Source: three-view drawing plus pictorial views. Frame: mm from the lowest corner of the part. A direction names the side the tool comes from. Give positions to 0.01 mm unless a question says otherwise; leave off trailing zeros. Write each loop counter-clockwise with the first axis right and the second up, starting at its lowest first coordinate (ties: lowest second). Pieces come first, ordered by that corner, then holes.
Q1. Pin query (flat end, axial travel): pin 1 (2.5 mm diameter, centred on x = 3.05, y = 4.5, fed in from +Z); pin 2 (3 mm diameter, centred on x = 13.5, y = 5, fed in from +Z); pin 3 (0.9 mm diameter, centred on x = 17, y = 6, fed in from -Z); pin 4 (1 mm diameter, centred on y = 3.5, z = 5.5, fed in from -X). Return the tip coordinate at first contact, or that it passes through.
Q2. Line query: L1, parallel to Y at x = 9, z = 4.2; L2, parallel to X at y = 3, z = 4.25; L3, parallel to Y at x = 12.25, z = 0.5. Output: solid intervals per line, ascending.
Q3. Cut plane B-B on z = 1.75. Return the cut outline in (x, y), plus the area to 3 significant figures.
Q4. Cut plane A-A on y = 4.5. Return the cut outline in (x, z), plus the area to 3 significant figures.
Q5. Cut plane D-D on x = 12.5. Return the cut outline in (y, z).
Q6. Draft query along Y for the marked faces 4, 5, 6 and 7. Return one class per face: pulls with the +Y half, pulls with the -Y half, needs draft (parallel to the pull), parting line crosses it, or undercut.
Q7. Cut plane C-C on y = 6. Return the cut outline in (x, z).
Q8. Reachability of the marked faces 1, 2 and 3 from +Z, -Z, +X, -X, +Y, -Y: full face, straight path, thin tool, end or side. Return the list, or none.
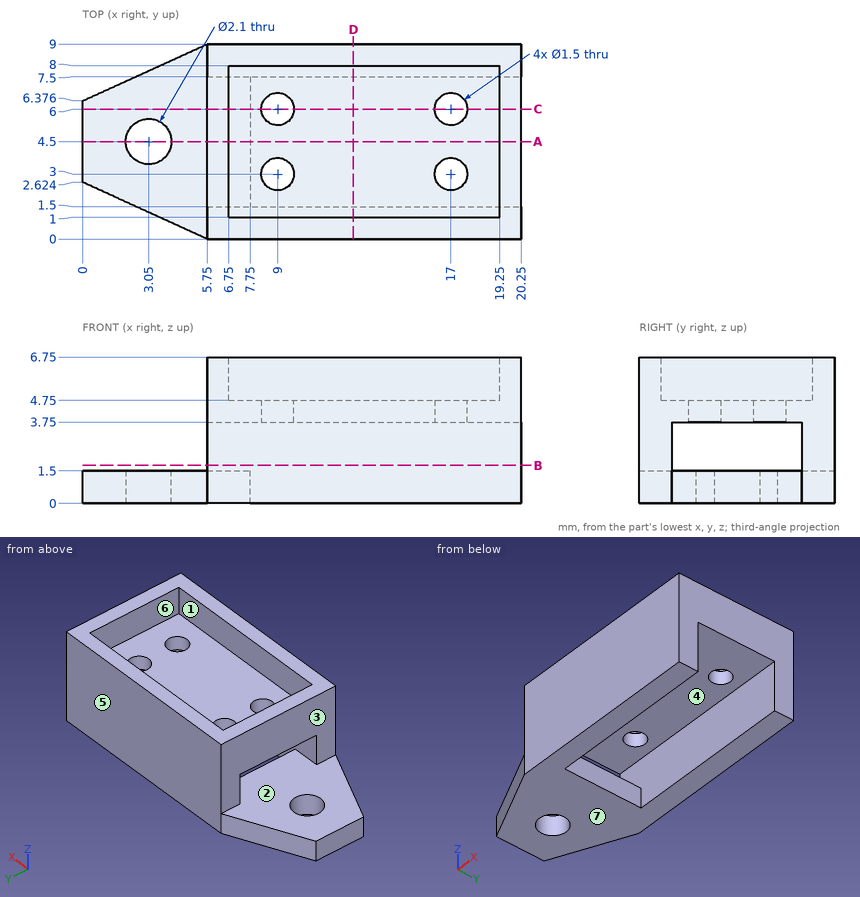
Data:
1. pin 1: stops at z = 1.5
1. pin 2: stops at z = 4.75
1. pin 3: passes through
1. pin 4: stops at x = 5.75
2. L1: y = 0 to 2.25, 3.75 to 5.25, 6.75 to 9
2. L2: x = 5.75 to 8.25, 9.75 to 16.25, 17.75 to 20.25
2. L3: y = 0 to 1.5, 7.5 to 9
3. outline: (5.75, 0) - (20.25, 0) - (20.25, 1.5) - (5.75, 1.5) - close; (5.75, 7.5) - (20.25, 7.5) - (20.25, 9) - (5.75, 9) - close
3. area: 43.5 mm2
4. outline: (0, 0) - (2, 0) - (2, 1.5) - (0, 1.5) - close; (4.1, 0) - (7.75, 0) - (7.75, 1.5) - (4.1, 1.5) - close; (5.75, 3.75) - (20.25, 3.75) - (20.25, 6.75) - (19.25, 6.75) - (19.25, 4.75) - (6.75, 4.75) - (6.75, 6.75) - (5.75, 6.75) - close
4. area: 27.0 mm2
5. outline: (0, 0) - (1.5, 0) - (1.5, 3.75) - (7.5, 3.75) - (7.5, 0) - (9, 0) - (9, 6.75) - (8, 6.75) - (8, 4.75) - (1, 4.75) - (1, 6.75) - (0, 6.75) - close
6. face 4: undercut
6. face 5: pulls with the +Y half
6. face 6: undercut
6. face 7: needs draft
7. outline: (0, 0) - (7.75, 0) - (7.75, 1.5) - (0, 1.5) - close; (5.75, 3.75) - (8.25, 3.75) - (8.25, 4.75) - (6.75, 4.75) - (6.75, 6.75) - (5.75, 6.75) - close; (9.75, 3.75) - (16.25, 3.75) - (16.25, 4.75) - (9.75, 4.75) - close; (17.75, 3.75) - (20.25, 3.75) - (20.25, 6.75) - (19.25, 6.75) - (19.25, 4.75) - (17.75, 4.75) - close
8. face 1: +Z
8. face 2: -X
8. face 3: +Z, -X, +Y, -Y
